Check sheet for the drawn part. Datum: minimum x, y, z corner. Units: mm. Give positions to 0.01 mm unless a question says otherwise; leave off trailing zeros. Write each loop counter-clockwise with the first axis right and the second up, starting at its lowest first coordinate (ties: lowest second). Pieces come first, ordered by that corner, then holes. Notation, with made-up numbers: M 14.5,74.25 L 65.5,74.25 A34 ccw 65.5,113.25 Z; hole C -20,-18 d8. An arc over 180 degrees is marked long. Write item = value, one per line.
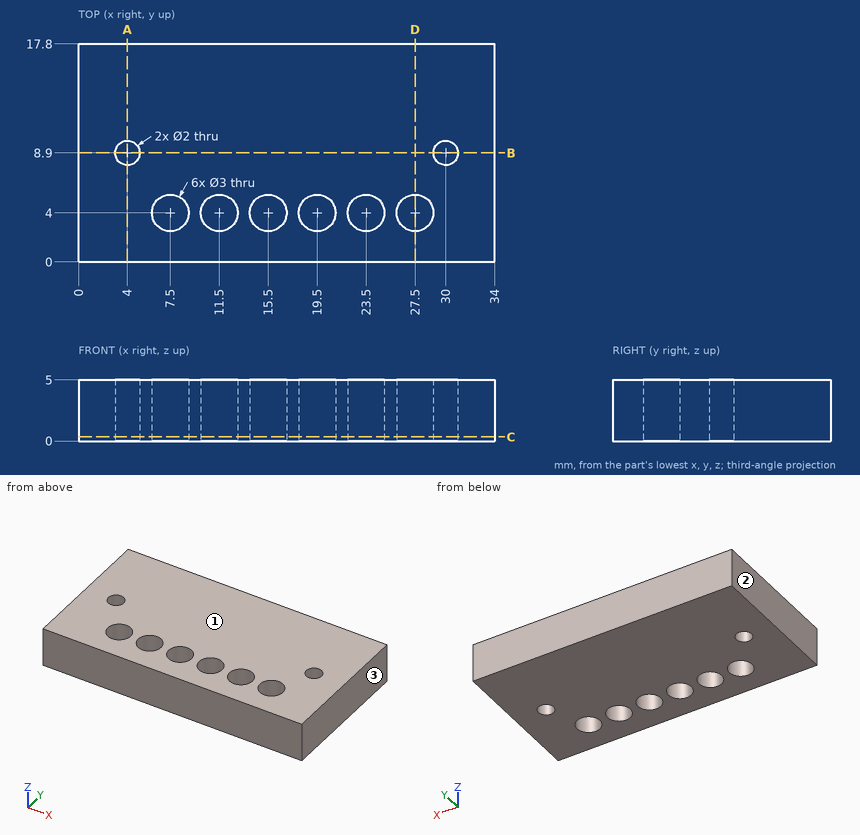
1) Draft check along X on the marked faces 1, 2 and 3. Enter one of: +X half, -X half, draft (parallel to the pull), parting line (faces both ways), or undercut.
From the geometry:
face_1 = draft
face_2 = -X half
face_3 = +X half
2) Cross-section at A-A on x = 4. Record the boundary of the cut face in (y, z).
From the geometry:
outline = M 0,0 L 7.9,0 L 7.9,5 L 0,5 Z; M 9.9,0 L 17.8,0 L 17.8,5 L 9.9,5 Z
3) Cross-section at B-B on y = 8.9. Record the boundary of the cut face in (x, z).
From the geometry:
outline = M 0,0 L 3,0 L 3,5 L 0,5 Z; M 5,0 L 29,0 L 29,5 L 5,5 Z; M 31,0 L 34,0 L 34,5 L 31,5 Z
4) Cross-section at D-D on x = 27.5. Record the boundary of the cut face in (y, z).
From the geometry:
outline = M 0,0 L 2.5,0 L 2.5,5 L 0,5 Z; M 5.5,0 L 17.8,0 L 17.8,5 L 5.5,5 Z
5) Cross-section at C-C on z = 0.35. Count the separate pieces of the cut face and the enclosed holes in it, plus the area to 3 significant figures.
From the geometry:
separate_pieces = 1
enclosed_holes = 8
area = 557 mm^2
6) Material ranges on probe 1 along Y at (x, z) = (27.5, 2.1); probe 2 along Y at (x, z) = (20, 1.8); probe 3 along X at (y, z) = (9.25, 2.35), recorded low to high. Write a range as from..to.
From the geometry:
probe_1 = 0..2.5, 5.5..17.8
probe_2 = 0..2.59, 5.41..17.8
probe_3 = 0..3.06, 4.94..29.06, 30.94..34
